Here's how the part is built. I have some questions about the finished solid (model axes, mm). Face numbers are marked on the shaded views. A direction names the side the tool comes from. Round coordinates to 2 decimals unless told otherwise and drop trailing zeros. Loops run counter-clockwise (first coordinate to the right, second up) from the corner with the lowest first, then second, coordinate; pieces in that order, holes last. Notation, with made-up numbers: (-18, 77.5) -> (1, 77.5) arc R16 cw to (1, 101.5) -> close; hole circle Ø4 at (73.5, 60). An arc over 180 degrees is marked (long way). Use CSV: the item, a comma, the result in double quotes. Start each with the question number.
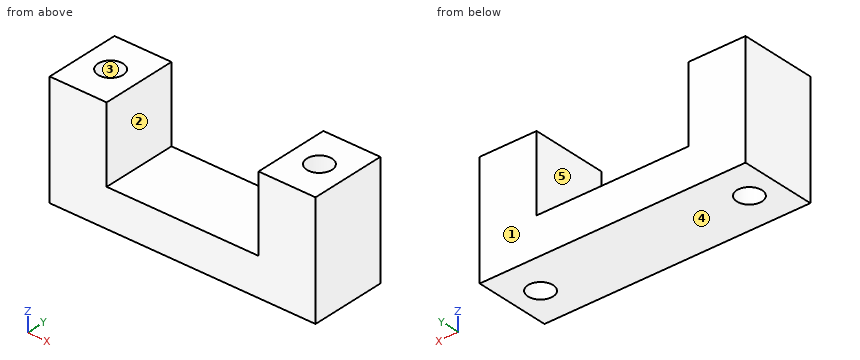
from build123d import *

# Parameters (mm, degrees)
SKETCH1_W           = 35
SKETCH1_H           = 10
SKETCH1_R           = 1.65
BOSS_EXTRUDE1_DEPTH = 15
SKETCH2_W           = 20
SKETCH2_H           = 10
CUT_EXTRUDE1_DEPTH  = 10


with BuildPart() as part:
    # Sketch1 → Boss-Extrude1 (new body)
    with BuildSketch(Plane.XY):
        Rectangle(SKETCH1_W, SKETCH1_H)
        with Locations((-13.75, 0)):
            Circle(SKETCH1_R, mode=Mode.SUBTRACT)
        with Locations((13.75, 0)):
            Circle(SKETCH1_R, mode=Mode.SUBTRACT)
    extrude(amount=BOSS_EXTRUDE1_DEPTH)

    # Sketch2 → Cut-Extrude1 (cut)
    with BuildSketch(Plane.XY.offset(15)):
        Rectangle(SKETCH2_W, SKETCH2_H)
    extrude(amount=-CUT_EXTRUDE1_DEPTH, mode=Mode.SUBTRACT)


solid = part.part
Q1. I want a section at A-A, the plane z = 11.5. List the corners of the cut face in (x, y) for me, then the cut area to 3 significant figures.
Q2. I want a section at D-D, the plane y = 2.75. List the corners of the cut face in (x, z) for me, then the cut area to 3 significant figures.
Q3. For the marked faces 4 and 5, which set-ups out of +Z, -Z, +X, -X, +Y, -Y let a thin tool reach every point of the face, with its end or its side?
Q4. I want a section at B-B, the plane x = 13.75. List the corners of the cut face in (y, z) for me.
Q5. Will these pins go through, and if not, where does the flat tip stop? pin 1 Ø5 at (x, y) = (4.5, 1.5) entering from +Z; pin 2 Ø2.5 at (x, y) = (13.75, 0) entering from +Z.
Q6. I want a section at C-C, the plane y = 0. List the corners of the cut face in (x, z) for me, then the cut area to 3 significant figures.
Q7. If we mould it in two halves opening along Y, with no side actions, what happens to the marked faces 1, 2 and 3? For each: pulls with the +Y half, pulls with the -Y half, needs draft (parallel to the pull), parting line crosses it, or undercut.
Q8. I need wall thicknesses on line 1 along X through (y, z) = (-3, 12.5); line 2 along Y through (x, z) = (13.75, 5.25); line 3 along X through (y, z) = (0.75, 13.75). Which ranges of each line are inside material? Lowest first, please.
Values found:
1,outline,"(-17.5, -5) -> (-10, -5) -> (-10, 5) -> (-17.5, 5) -> close; (10, -5) -> (17.5, -5) -> (17.5, 5) -> (10, 5) -> close; hole circle Ø3.3 at (-13.75, 0); hole circle Ø3.3 at (13.75, 0)"
1,area,"133 mm2"
2,outline,"(-17.5, 0) -> (17.5, 0) -> (17.5, 15) -> (10, 15) -> (10, 5) -> (-10, 5) -> (-10, 15) -> (-17.5, 15) -> close"
2,area,"325 mm2"
3,face 4,"-Z, +X, -X, +Y, -Y"
3,face 5,"+Z, +Y, -Y"
4,outline,"(-5, 0) -> (-1.65, 0) -> (-1.65, 15) -> (-5, 15) -> close; (1.65, 0) -> (5, 0) -> (5, 15) -> (1.65, 15) -> close"
5,pin 1,"z = 5"
5,pin 2,"through"
6,outline,"(-17.5, 0) -> (-15.4, 0) -> (-15.4, 15) -> (-17.5, 15) -> close; (-12.1, 0) -> (12.1, 0) -> (12.1, 15) -> (10, 15) -> (10, 5) -> (-10, 5) -> (-10, 15) -> (-12.1, 15) -> close; (15.4, 0) -> (17.5, 0) -> (17.5, 15) -> (15.4, 15) -> close"
6,area,"226 mm2"
7,face 1,"pulls with the +Y half"
7,face 2,"needs draft"
7,face 3,"undercut"
8,line 1,"-17.5 to -10, 10 to 17.5"
8,line 2,"-5 to -1.65, 1.65 to 5"
8,line 3,"-17.5 to -15.22, -12.28 to -10, 10 to 12.28, 15.22 to 17.5"
